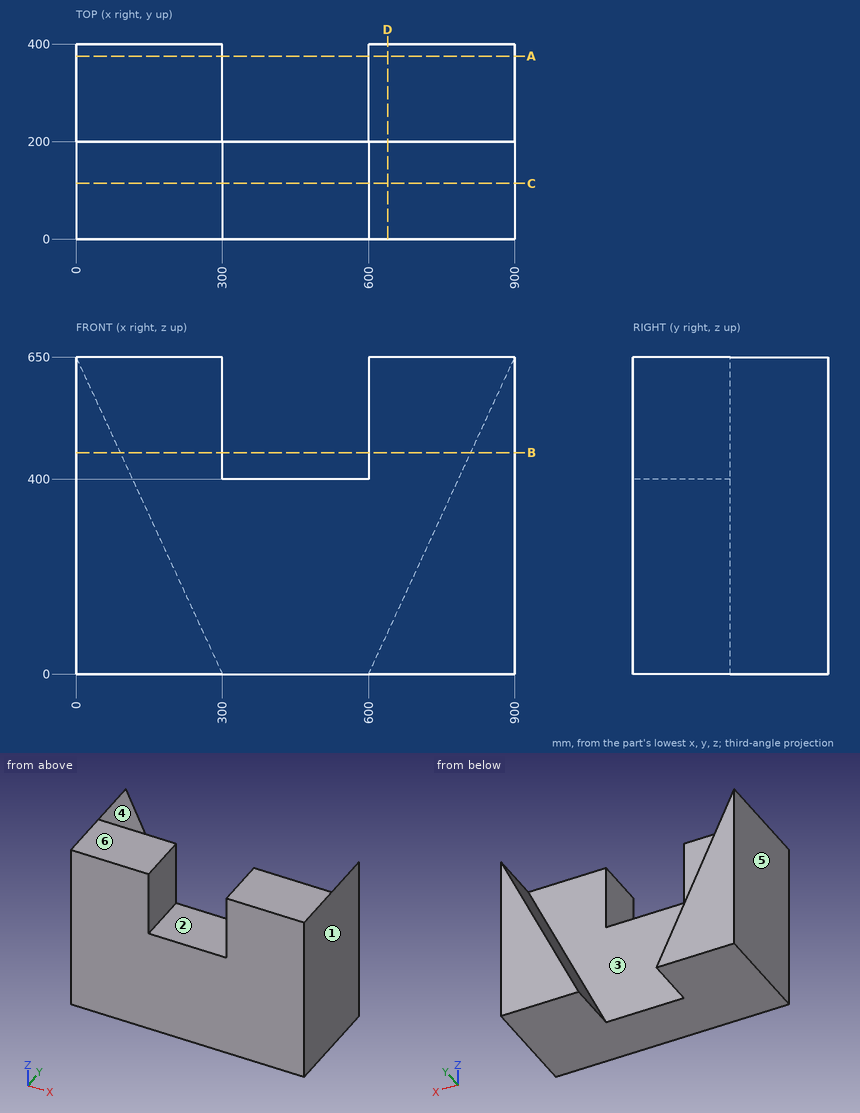
Check sheet for the drawn part. Datum: minimum x, y, z corner. Units: mm. A direction names the side the tool comes from. Round coordinates to 2 decimals unless told otherwise and drop trailing zeros. Loops run counter-clockwise (first coordinate to the right, second up) from the corner with the lowest first, then second, coordinate; pieces in that order, holes last. Notation, with made-up numbers: (61, 13.5) - (65, 13.5) arc R16 cw to (65, 35.5) - close; hole circle Ø10 at (-32, 55). An arc over 180 degrees is marked (long way). Write item = value, one per line. Start each with the question number.
1. Section check A-A on y = 375. Enter the section's corners in (x, z).
2. Depth check by flat-ended pin: pin 1 (5 mm diameter, centred on x = 210, z = 433.5, fed in from +Y); pin 2 (1.5 mm diameter, centred on y = 57, z = 315.5, fed in from -X); pin 3 (4 mm diameter, centred on x = 600.5, y = 295, fed in from +Z). Enter the tip coordinate at first touch or a pass-through.
3. Section check C-C on y = 114. Enter the section's corners in (x, z), then the cut area to 3 significant figures.
4. Mould release check, pull along X, two halves, no side actions. Record for the marked faces 3, 4, 5 and 6: released by +X, released by -X, zero draft, split by the parting line, or undercut.
5. Set-up check for the marked faces 1 and 2: record each of +Z, -Z, +X, -X, +Y, -Y from which the full face is reachable in a straight line by a thin tool's end or side.
6. Thickness scan on line 1 (Y direction, x = 234.5, z = 177); line 2 (X direction, y = 49, z = 465); line 3 (Z direction, x = 356.5, y = 66). Record the ranges inside material, lowest first.
7. Section check D-D on x = 639. Enter the section's corners in (y, z), then the cut area to 3 significant figures.
8. Section check B-B on z = 454. Enter the section's corners in (x, y), then the cut area to 3 significant figures.
Working result:
q1.outline = (0, 0) - (300, 0) - (0, 650) - close; (600, 0) - (900, 0) - (900, 650) - close
q2.pin_1 = 200
q2.pin_2 = 0
q2.pin_3 = 5.42
q3.outline = (0, 0) - (900, 0) - (900, 650) - (600, 650) - (600, 400) - (300, 400) - (300, 650) - (0, 650) - close
q3.area = 510,000 mm^2
q4.face_3 = undercut
q4.face_4 = undercut
q4.face_5 = released by -X
q4.face_6 = zero draft
q5.face_1 = +Z, -Z, +X, +Y, -Y
q5.face_2 = +Z, +Y, -Y
q6.line_1 = 0 to 200
q6.line_2 = 0 to 300, 600 to 900
q6.line_3 = 0 to 400
q7.outline = (0, 0) - (400, 0) - (400, 84.5) - (200, 84.5) - (200, 650) - (0, 650) - close
q7.area = 147,000 mm^2
q8.outline = (0, 0) - (300, 0) - (300, 200) - (90.46, 200) - (90.46, 400) - (0, 400) - close; (600, 0) - (900, 0) - (900, 400) - (809.54, 400) - (809.54, 200) - (600, 200) - close
q8.area = 156,000 mm^2
